Geometry: final body of the model. Coordinates: model frame, mm. A direction names the side the tool comes from. Coordinates: 2 decimals unless noted, no trailing zeros. Order: outer loops, then holes, each group sorted by start corner. A loop starts at its lowest first (then second) coordinate and runs counter-clockwise, first axis right, second up. Notation, with made-up numbers: (64.5, 80.25) -> (119.5, 80.25) arc R26 cw to (119.5, 104.25) -> close; hole circle Ø8 at (10.25, -5). An arc over 180 degrees is marked (long way). Answer in a Markdown table with one row per item. Add a question column.
1) Ray query, line 1 (X direction, y = 5, z = 5); line 2 (Z direction, x = 2.75, y = 6.25); line 3 (Z direction, x = 5, y = 5). Return the intervals inside material, ascending. Write a range as from..to.
2) Pull-direction query (Z, two-part tool) for faces 1 (the face through (10, 5, 0)), 2 (the face through (8, 4, 3)), 3 (the face through (3.8, 6.2, 8.1)); classes: +Z half, -Z half, draft (parallel to the pull), parting line (faces both ways), or undercut.
3) Set-up query: faces 4 (the face through (8, 0, 7)), 5 (the face through (2.89, 3.84, 8.9)), 6 (the face through (3, 1, 5.49)). Return all of +Z, -Z, +X, -X, +Y, -Y with unobstructed straight access to the full face (end or side cutting, diameter ignored); none if empty.
4) Section query B-B on z = 1.25. Return the cut outline in (x, y), then the cut area to 3 significant figures.
5) Section query A-A on y = 9.5. Return the cut outline in (x, z).
6) Section query D-D on y = 5.5. Return the cut outline in (x, z), then the cut area to 3 significant figures.
7) Section query C-C on x = 6. Return the cut outline in (y, z).
```python
from build123d import *

# Parameters (mm, degrees)
SKETCH2_W           = 16.23
SKETCH2_H           = 10
SKETCH2_R           = 1.5
BOSS_EXTRUDE1_DEPTH = 13.7
SKETCH3_R           = 1.5
CUT_EXTRUDE1_DEPTH  = 24.47558093
CUT_EXTRUDE4_DEPTH  = 1.8
SKETCH7_W           = 1.8
SKETCH7_H           = 5.438639536
CUT_EXTRUDE5_DEPTH  = 5
SKETCH8_W           = 1.8
SKETCH8_H           = 2.719319768
CUT_EXTRUDE6_DEPTH  = 23.476630642


with BuildPart() as part:
    # Sketch2 → Boss-Extrude1 (new body)
    with BuildSketch(Plane.XY):
        with Locations((8.115, 5)):
            Rectangle(SKETCH2_W, SKETCH2_H)
        with Locations(Location((6.882853167, 5, 0), (0, 0, 180))):
            Circle(SKETCH2_R, mode=Mode.SUBTRACT)
    extrude(amount=BOSS_EXTRUDE1_DEPTH)

    # Sketch3 → Cut-Extrude1 (cut, through all)
    with BuildSketch(Plane(origin=(16.23, 0, 0), x_dir=(0, 0, -1), z_dir=(1, 0, 0))):
        with Locations((-6.85, 5)):
            Circle(SKETCH3_R)
    extrude(amount=-CUT_EXTRUDE1_DEPTH, mode=Mode.SUBTRACT)

    # Sketch4 → Cut-Extrude4 (cut)
    with BuildSketch(Plane(origin=(2, 0, 0), x_dir=(0, 0, -1), z_dir=(1, 0, 0))):
        Polygon((-5.490340116, 2.645), (-4.130680232, 5), (-5.490340116, 7.355), (-8.209659884, 7.355), (-9.569319768, 5), (-8.209659884, 2.645), align=None)
    extrude(amount=CUT_EXTRUDE4_DEPTH, mode=Mode.SUBTRACT)

    # Sketch7 → Cut-Extrude5 (cut)
    with BuildSketch(Plane(origin=(0, 10, 0), x_dir=(1, 0, 0), z_dir=(0, 1, 0))):
        with Locations((2.9, -6.85)):
            Rectangle(SKETCH7_W, SKETCH7_H)
    extrude(amount=-CUT_EXTRUDE5_DEPTH, mode=Mode.SUBTRACT)

    # Sketch8 → Cut-Extrude6 (cut, through all)
    with BuildSketch(Plane(origin=(0, 2.645, 0), x_dir=(1, 0, 0), z_dir=(0, 1, 0))):
        with Locations((2.9, -6.85)):
            Rectangle(SKETCH8_W, SKETCH8_H)
    extrude(amount=-CUT_EXTRUDE6_DEPTH, mode=Mode.SUBTRACT)


solid = part.part
```
Result:
| question | item | result |
|---|---|---|
| 1 | line 1 | 0..2, 3.8..5.38, 8.38..16.23 |
| 1 | line 2 | 0..4.13, 9.57..13.7 |
| 1 | line 3 | 0..5.35, 8.35..13.7 |
| 2 | face 1 | -Z half |
| 2 | face 2 | draft |
| 2 | face 3 | undercut |
| 3 | face 4 | +Z, -Z, +X, -X, -Y |
| 3 | face 5 | +Y |
| 3 | face 6 | +Y, -Y |
| 4 | outline | (0, 0) -> (16.23, 0) -> (16.23, 10) -> (0, 10) -> close; hole circle Ø3 at (6.88, 5) |
| 4 | area | 155 mm2 |
| 5 | outline | (0, 0) -> (16.23, 0) -> (16.23, 13.7) -> (0, 13.7) -> close; hole (2, 4.13) -> (3.8, 4.13) -> (3.8, 9.57) -> (2, 9.57) -> close |
| 6 | outline | (0, 0) -> (5.47, 0) -> (5.47, 5.44) -> (3.8, 5.44) -> (3.8, 4.13) -> (2, 4.13) -> (2, 5.44) -> (0, 5.44) -> close; (0, 8.26) -> (2, 8.26) -> (2, 9.57) -> (3.8, 9.57) -> (3.8, 8.26) -> (5.47, 8.26) -> (5.47, 13.7) -> (0, 13.7) -> close; (8.3, 0) -> (16.23, 0) -> (16.23, 5.44) -> (8.3, 5.44) -> close; (8.3, 8.26) -> (16.23, 8.26) -> (16.23, 13.7) -> (8.3, 13.7) -> close |
| 6 | area | 141 mm2 |
| 7 | outline | (0, 0) -> (3.79, 0) -> (3.79, 5.97) arc R1.5 cw to (3.79, 7.73) -> (3.79, 13.7) -> (0, 13.7) -> close; (6.21, 0) -> (10, 0) -> (10, 13.7) -> (6.21, 13.7) -> (6.21, 7.73) arc R1.5 cw to (6.21, 5.97) -> close |
